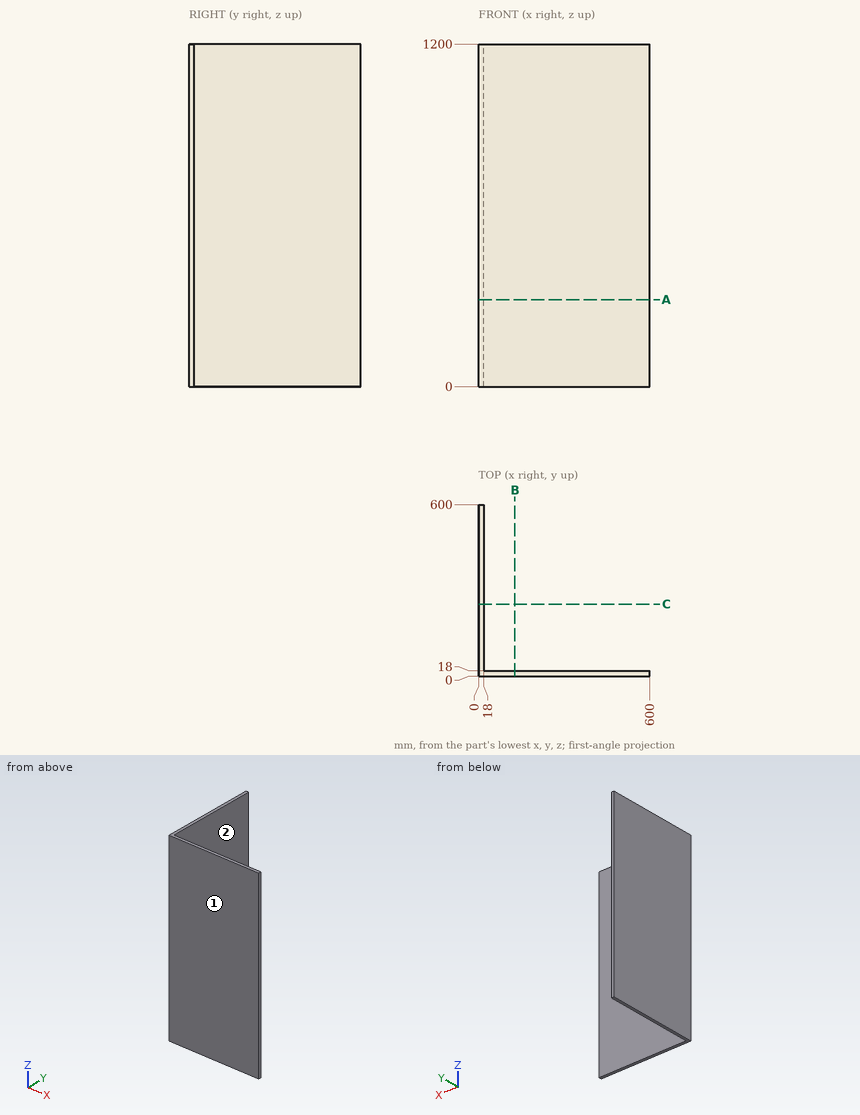
Print and shaded views of the part. All mm, measured from the part's lowest x, y and z. A direction names the side the tool comes from. Round coordinates to 2 decimals unless told otherwise and drop trailing zeros. Loops run counter-clockwise (first coordinate to the right, second up) from the corner with the lowest first, then second, coordinate; pieces in that order, holes last. Notation, with made-up numbers: (31.25, 18) -> (42.25, 18) arc R27 ccw to (42.25, 38) -> close; hole circle Ø7 at (83, 75). An arc over 180 degrees is marked (long way). Use CSV: the item, a comma, the result in double quotes. Start each with the question number.
1) Which spindle directions (+Z, -Z, +X, -X, +Y, -Y) get a long thin tool onto all of the face, cutting with end or side? Do the marked faces 1 and 2. Say none if no direction does.
2) Drop flat-ended pins along their axis: P1, Ø5, axis at x = 262.5, z = 128, coming from the -Y side; P2, Ø1, axis at y = 202, z = 832.5, coming from the +X side; P3, Ø2, axis at x = 516, z = 260, coming from the +Y side. Give the stop position or say it passes through.
3) Wall check: L1, parallel to Y at x = 472.5, z = 413. Give the ranges that are in metal, low to high. Write a range as [from, to].
4) Cut at B-B, the plane x = 127. Write the cut outline in (y, z), plus the area to 3 significant figures.
5) Cut at A-A, the plane z = 305. Write the cut outline in (x, y), plus the area to 3 significant figures.
Determined:
1,face 1,"+Z, -Z, +X, -X, -Y"
1,face 2,"+Z, -Z, +X, +Y"
2,P1,"stops at y = 0"
2,P2,"stops at x = 18"
2,P3,"stops at y = 18"
3,L1,"y = [0, 18]"
4,outline,"(0, 0) -> (18, 0) -> (18, 1200) -> (0, 1200) -> close"
4,area,"21,600 mm2"
5,outline,"(0, 0) -> (600, 0) -> (600, 18) -> (18, 18) -> (18, 600) -> (0, 600) -> close"
5,area,"21,300 mm2"
